CAD build for the part. Positions are in the model's coordinates, mm. Face numbers are marked on the shaded views. A direction names the side the tool comes from. Coordinates: 2 decimals unless noted, no trailing zeros. Loops run counter-clockwise (first coordinate to the right, second up) from the corner with the lowest first, then second, coordinate; pieces in that order, holes last.
1) Two-plate mould, pull along Z, no slides. Class the marked faces 1, 2 and 3: +Z half, -Z half, draft (parallel to the pull), parting line (faces both ways), or undercut.
2) Saw through at B-B, the plane x = 4.5. Write the cut outline in (y, z).
3) Pin check, flat tips, straight feed: pin 1 Ø1.4 at (x, y) = (6, 32.5) entering from +Z; pin 2 Ø4 at (y, z) = (26.5, 12) entering from +X; pin 3 Ø1.5 at (x, z) = (9, 12.5) entering from +Y. Stop position of each tip, or through.
4) Wall check: line 1 along Z through (x, y) = (1.5, 12.5); line 2 along Z through (x, y) = (7, 32.5); line 3 along Y through (x, z) = (14, 1.25). Give the ranges that are in metal, low to high.
5) Which spindle directions (+Z, -Z, +X, -X, +Y, -Y) get a long thin tool onto all of the face, cutting with end or side? Do the marked faces 4, 5, 6, 7 and 8. Say none if no direction does.
6) Saw through at C-C, the plane z = 7.75. Give the number of separate pieces and of enclosed holes in the cut face, and give its area (3 significant figures).
7) Saw through at A-A, the plane z = 23.25. Write the cut outline in (x, y), and give its area (3 significant figures).
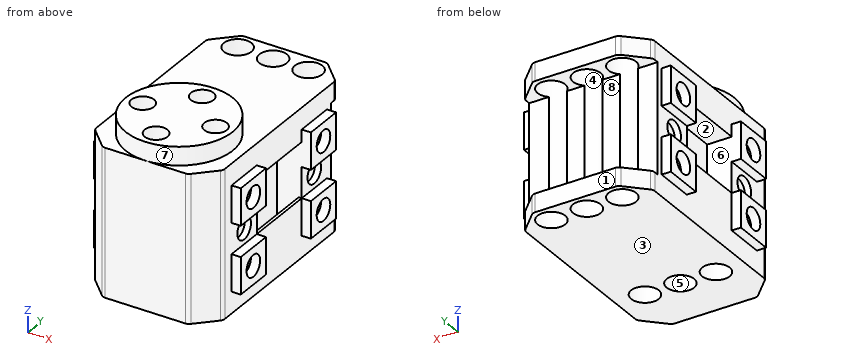
```python
from build123d import *

# Parameters (mm, degrees)
BOSS_EXTRU_1_DEPTH           = 24
CONG_1_R                     = 1
ESQUISSE2_W                  = 6
ESQUISSE2_H                  = 6.5
ESQUISSE2_R                  = 1.75
BOSS_EXTRU_2_DEPTH           = 1.5
ENL_V_MAT_EXTRU_1_DEPTH      = 45.775212404
ENL_V_MAT_EXTRU_1_DEPTH_BACK = 45.775212404
ESQUISSE4_W                  = 18
ESQUISSE4_H                  = 4.7
ESQUISSE5_R                  = 2.25
ENL_V_MAT_EXTRU_2_DEPTH      = 49.494179566
ESQUISSE6_W                  = 9
ESQUISSE6_H                  = 11.6
ENL_V_MAT_EXTRU_3_DEPTH      = 4
ESQUISSE7_R                  = 1.75
ENL_V_MAT_EXTRU_4_DEPTH      = 1
ESQUISSE8_R                  = 8.75
ESQUISSE8_R_2                = 1.85
BOSS_EXTRU_3_DEPTH           = 3
ESQUISSE9_W                  = 3.5
ESQUISSE9_H                  = 11.6
ENL_V_MAT_EXTRU_5_DEPTH      = 4.5
ESQUISSE10_R                 = 2.25
ENL_V_MAT_EXTRU_6_DEPTH      = 3


with BuildPart() as part:
    # Esquisse1 → Boss.-Extru.1 (new body)
    with BuildSketch(Plane.XY):
        Polygon((3.191025459, -0.155619048), (-0.344508447, 3.379914858), (-0.344508447, 32.308847046), (3.191025459, 35.844380952), (17.119957647, 35.844380952), (20.655491553, 32.308847046), (20.655491553, 3.379914858), (17.119957647, -0.155619048), align=None)
    extrude(amount=BOSS_EXTRU_1_DEPTH)

    # Congé1
    cong_1_edges = [part.edges().sort_by_distance(p)[0] for p in [
        (3.191025459, -0.155619048, 12),
        (-0.344508447, 3.379914858, 12),
        (-0.344508447, 32.308847046, 12),
        (3.191025459, 35.844380952, 12),
        (17.119957647, 35.844380952, 12),
        (20.655491553, 32.308847046, 12),
        (20.655491553, 3.379914858, 12),
        (17.119957647, -0.155619048, 12),
    ]]
    fillet(cong_1_edges, radius=CONG_1_R)

    # Esquisse2 → Boss.-Extru.2 (add)
    # profile 1 of 4: a face of its own
    with BuildSketch(Plane(origin=(20.655491553, 0, 0), x_dir=(0, 0, -1), z_dir=(1, 0, 0))):
        with Locations((-17.5, 8.794380952)):
            Rectangle(ESQUISSE2_W, ESQUISSE2_H)
        with Locations(Location((-17.5, 8.794380952, 0), (0, 0, 90))):
            Circle(ESQUISSE2_R, mode=Mode.SUBTRACT)
    # profile 2 of 4: a face of its own
    with BuildSketch(Plane(origin=(20.655491553, 0, 0), x_dir=(0, 0, -1), z_dir=(1, 0, 0))):
        with Locations((-6.5, 8.794380952)):
            Rectangle(ESQUISSE2_W, ESQUISSE2_H)
        with Locations(Location((-6.5, 8.794380952, 0), (0, 0, 90))):
            Circle(ESQUISSE2_R, mode=Mode.SUBTRACT)
    # profile 3 of 4: a face of its own
    with BuildSketch(Plane(origin=(20.655491553, 0, 0), x_dir=(0, 0, -1), z_dir=(1, 0, 0))):
        with Locations((-17.5, 26.894380952)):
            Rectangle(ESQUISSE2_W, ESQUISSE2_H)
        with Locations(Location((-17.5, 26.894380952, 0), (0, 0, 90))):
            Circle(ESQUISSE2_R, mode=Mode.SUBTRACT)
    # profile 4 of 4: a face of its own
    with BuildSketch(Plane(origin=(20.655491553, 0, 0), x_dir=(0, 0, -1), z_dir=(1, 0, 0))):
        with Locations((-6.5, 26.894380952)):
            Rectangle(ESQUISSE2_W, ESQUISSE2_H)
        with Locations(Location((-6.5, 26.894380952, 0), (0, 0, 90))):
            Circle(ESQUISSE2_R, mode=Mode.SUBTRACT)
    boss_extru_2 = extrude(amount=BOSS_EXTRU_2_DEPTH)

    # Symétrie1: Boss.-Extru.2 across plane
    add(boss_extru_2.mirror(Plane(origin=(10.155491553, 0, 0), x_dir=(0, 0, 1), z_dir=(1, 0, 0))))

    # Esquisse4 → Enlèv. mat.-Extru.1 (cut, two sides: drawn at the far end of the back side and taken through both)
    with BuildSketch(Plane(origin=(10.155491553, 0, 0), x_dir=(0, 0, -1), z_dir=(1, 0, 0)).offset(-ENL_V_MAT_EXTRU_1_DEPTH_BACK)):
        with Locations((-12, 33.494380952)):
            Rectangle(ESQUISSE4_W, ESQUISSE4_H)
    extrude(amount=ENL_V_MAT_EXTRU_1_DEPTH + ENL_V_MAT_EXTRU_1_DEPTH_BACK, mode=Mode.SUBTRACT)

    # Esquisse5 → Enlèv. mat.-Extru.2 (cut, through all)
    with BuildSketch(Plane.XY.offset(24)):
        with Locations((4.355491553, 32.844380952)):
            Circle(ESQUISSE5_R)
        with Locations((10.155491553, 32.844380952)):
            Circle(ESQUISSE5_R)
        with Locations((15.955491553, 32.844380952)):
            Circle(ESQUISSE5_R)
    extrude(amount=-ENL_V_MAT_EXTRU_2_DEPTH, mode=Mode.SUBTRACT)

    # Esquisse6 → Enlèv. mat.-Extru.3 (cut)
    with BuildSketch(Plane(origin=(20.655491553, 0, 0), x_dir=(0, 0, -1), z_dir=(1, 0, 0))):
        with Locations((-14, 17.844380952)):
            Rectangle(ESQUISSE6_W, ESQUISSE6_H)
    enl_v_mat_extru_3 = extrude(amount=-ENL_V_MAT_EXTRU_3_DEPTH, mode=Mode.SUBTRACT)

    # Symétrie2: Enlèv. mat.-Extru.3 across plane
    add(enl_v_mat_extru_3.mirror(Plane(origin=(10.155491553, 0, 0), x_dir=(0, 0, 1), z_dir=(1, 0, 0))), mode=Mode.SUBTRACT)

    # Esquisse7 → Enlèv. mat.-Extru.4 (cut)
    with BuildSketch(Plane(origin=(20.655491553, 0, 0), x_dir=(0, 0, -1), z_dir=(1, 0, 0))):
        with Locations(Location((-12, 8.794380952, 0), (0, 0, 90))):
            Circle(ESQUISSE7_R)
        with Locations(Location((-12, 26.894380952, 0), (0, 0, 90))):
            Circle(ESQUISSE7_R)
    enl_v_mat_extru_4 = extrude(amount=-ENL_V_MAT_EXTRU_4_DEPTH, mode=Mode.SUBTRACT)

    # Symétrie3: Enlèv. mat.-Extru.4 across plane
    add(enl_v_mat_extru_4.mirror(Plane(origin=(10.155491553, 0, 0), x_dir=(0, 0, 1), z_dir=(1, 0, 0))), mode=Mode.SUBTRACT)

    # Esquisse8 → Boss.-Extru.3 (add)
    with BuildSketch(Plane.XY.offset(24)):
        with Locations(Location((10.155491553, 8.594380952, 0), (0, 0, 270))):
            Circle(ESQUISSE8_R)
        with Locations((10.155491553, 2.644380952)):
            Circle(ESQUISSE8_R_2, mode=Mode.SUBTRACT)
        with Locations((4.205491553, 8.594380952)):
            Circle(ESQUISSE8_R_2, mode=Mode.SUBTRACT)
        with Locations((10.155491553, 14.544380952)):
            Circle(ESQUISSE8_R_2, mode=Mode.SUBTRACT)
        with Locations((16.105491553, 8.594380952)):
            Circle(ESQUISSE8_R_2, mode=Mode.SUBTRACT)
    extrude(amount=BOSS_EXTRU_3_DEPTH)

    # Esquisse9 → Enlèv. mat.-Extru.5 (cut)
    with BuildSketch(Plane.XY.offset(9.5)):
        with Locations((18.405491553, 17.844380952)):
            Rectangle(ESQUISSE9_W, ESQUISSE9_H)
    enl_v_mat_extru_5 = extrude(amount=-ENL_V_MAT_EXTRU_5_DEPTH, mode=Mode.SUBTRACT)

    # Symétrie4: Enlèv. mat.-Extru.5 across plane
    add(enl_v_mat_extru_5.mirror(Plane(origin=(10.155491553, 0, 0), x_dir=(0, 0, 1), z_dir=(1, 0, 0))), mode=Mode.SUBTRACT)

    # Esquisse10 → Enlèv. mat.-Extru.6 (cut)
    with BuildSketch(Plane(origin=(0, 0, 0), x_dir=(-1, 0, 0), z_dir=(0, 0, -1))):
        with Locations((-10.155491553, 8.694380952)):
            Circle(ESQUISSE10_R)
        with Locations((-15.955491553, 8.694380952)):
            Circle(ESQUISSE10_R)
        with Locations((-4.355491553, 8.694380952)):
            Circle(ESQUISSE10_R)
    extrude(amount=-ENL_V_MAT_EXTRU_6_DEPTH, mode=Mode.SUBTRACT)


solid = part.part
```
Data:
1. face 1: draft
1. face 2: undercut
1. face 3: -Z half
2. outline: (-0.16, 0) - (6.45, 0) - (6.45, 3) - (10.94, 3) - (10.94, 0) - (30.6, 0) - (30.6, 24) - (15.27, 24) - (15.27, 27) - (10.42, 27) - (10.42, 24) - (6.77, 24) - (6.77, 27) - (1.92, 27) - (1.92, 24) - (-0.16, 24) - close; (35.09, 0) - (35.84, 0) - (35.84, 3) - (35.09, 3) - close; (35.09, 21) - (35.84, 21) - (35.84, 24) - (35.09, 24) - close
3. pin 1: stops at z = 24
3. pin 2: stops at x = 20.66
3. pin 3: stops at y = 31.14
4. line 1: z = 0 to 5, 18.5 to 24
4. line 2: z = 0 to 3, 21 to 24
4. line 3: y = -0.16 to 7.58, 9.81 to 31.73, 33.96 to 35.84
5. face 4: +Z, -Z
5. face 5: -Z
5. face 6: none
5. face 7: +Z
5. face 8: +X, -X, +Y
6. separate pieces: 1
6. enclosed holes: 2
6. area: 584 mm2
7. outline: (-0.34, 3.79) arc R1 ccw to (-0.05, 3.09) - (2.9, 0.14) arc R1 ccw to (3.61, -0.16) - (16.71, -0.16) arc R1 ccw to (17.41, 0.14) - (20.36, 3.09) arc R1 ccw to (20.66, 3.79) - (20.66, 31.89) arc R1 ccw to (20.36, 32.6) - (17.41, 35.55) arc R1 ccw to (16.71, 35.84) - (3.61, 35.84) arc R1 ccw to (2.9, 35.55) - (-0.05, 32.6) arc R1 ccw to (-0.34, 31.89) - close; hole circle Ø4.5 at (4.36, 32.84); hole circle Ø4.5 at (10.16, 32.84); hole circle Ø4.5 at (15.96, 32.84)
7. area: 683 mm2
